Could you check a few things on this model? Use its own coordinates, in mm. A direction names the side the tool comes from. Round coordinates to 2 decimals unless told otherwise and drop trailing zeros. Write each loop counter-clockwise with the first axis right and the second up, starting at its lowest first coordinate (ties: lowest second). Pieces come first, ordered by that corner, then holes. Notation, with made-up numbers: (-7.5, 42) -> (15.5, 42) arc R11 cw to (15.5, 47) -> close; hole circle Ø10 at (17.5, 30). An arc over 180 degrees is marked (long way). Return JSON: item names as keys, results as strings.
from build123d import *

# Parameters (mm, degrees)
SKETCH_1_W      = 50
SKETCH_1_H      = 49
SKETCH_1_R      = 11.05
SKETCH_1_R_2    = 1.75
EXTRUDE_1_DEPTH = 2
EXTRUDE_2_DEPTH = 2
FILLET_2_R      = 2


with BuildPart() as part:
    # 草图1 → 凸台-拉伸1 (new body)
    with BuildSketch(Plane(origin=(0, 0, 0), x_dir=(1, 0, 0), z_dir=(0, 1, 0))):
        with Locations((-25, 0)):
            Rectangle(SKETCH_1_W, SKETCH_1_H)
        with Locations(Location((-25, 3.5, 0), (0, 0, 270))):
            Circle(SKETCH_1_R, mode=Mode.SUBTRACT)
        with Locations(Location((-40.5, 19, 0), (0, 0, 270))):
            Circle(SKETCH_1_R_2, mode=Mode.SUBTRACT)
        with Locations(Location((-9.5, 19, 0), (0, 0, 270))):
            Circle(SKETCH_1_R_2, mode=Mode.SUBTRACT)
        with Locations(Location((-9.5, -12, 0), (0, 0, 270))):
            Circle(SKETCH_1_R_2, mode=Mode.SUBTRACT)
        with Locations(Location((-40.5, -12, 0), (0, 0, 270))):
            Circle(SKETCH_1_R_2, mode=Mode.SUBTRACT)
    extrude(amount=EXTRUDE_1_DEPTH)

    # 草图2 → 凸台-拉伸2 (add)
    with BuildSketch(Plane.XY.offset(24.5)):
        Polygon((0, 0), (0, -51), (-50, -51), (-50, 0), (-50, 2), (0, 2), align=None)
        with BuildLine():
            Line((-7.9, -10), (-7.9, -40))
            ThreePointArc((-7.9, -40), (-10, -42.1), (-12.1, -40))
            Line((-12.1, -40), (-12.1, -10))
            ThreePointArc((-12.1, -10), (-10, -7.9), (-7.9, -10))
        make_face(mode=Mode.SUBTRACT)
        with BuildLine():
            Line((-37.9, -10), (-37.9, -40))
            ThreePointArc((-37.9, -40), (-40, -42.1), (-42.1, -40))
            Line((-42.1, -40), (-42.1, -10))
            ThreePointArc((-42.1, -10), (-40, -7.9), (-37.9, -10))
        make_face(mode=Mode.SUBTRACT)
    extrude(amount=EXTRUDE_2_DEPTH)

    # 圆角2
    fillet_2_edges = [part.edges().sort_by_distance(p)[0] for p in [
        (-25, 2, 26.5),
    ]]
    fillet(fillet_2_edges, radius=FILLET_2_R)


solid = part.part
1) I want a section at C-C, the plane y = -24. Please give me the cut outline in (x, z), and give its area (3 significant figures).
Return value:
{"outline": "(-50, 24.5) -> (-42.1, 24.5) -> (-42.1, 26.5) -> (-50, 26.5) -> close; (-37.9, 24.5) -> (-12.1, 24.5) -> (-12.1, 26.5) -> (-37.9, 26.5) -> close; (-7.9, 24.5) -> (0, 24.5) -> (0, 26.5) -> (-7.9, 26.5) -> close", "area": "83.2 mm²"}
2) I want a section at D-D, the plane z = 12. Please give me the cut outline in (x, y), and give its area (3 significant figures).
Return value:
{"outline": "(-50, 0) -> (-42.25, 0) -> (-42.25, 2) -> (-50, 2) -> close; (-38.75, 0) -> (-11.25, 0) -> (-11.25, 2) -> (-38.75, 2) -> close; (-7.75, 0) -> (0, 0) -> (0, 2) -> (-7.75, 2) -> close", "area": "86.0 mm²"}
3) For faces 5 (the face through (-40, -7.9, 25.5)), 6 (the face through (-25, 0, 11)), 7 (the face through (-24.65, 1.43, 25.9)), which set-ups out of +Z, -Z, +X, -X, +Y, -Y let a thin tool reach every point of the face, with its end or its side?
Return value:
{"face 5": "+Z, -Z", "face 6": "-Z, +X, -X, -Y", "face 7": "+Z, +X, -X, +Y"}
4) I want a section at B-B, the plane x = -25. Please give me the cut outline in (y, z).
Return value:
{"outline": "(-51, 24.5) -> (0, 24.5) -> (0, 7.55) -> (2, 7.55) -> (2, 24.5) arc R2 ccw to (0, 26.5) -> (-51, 26.5) -> close; (0, -24.5) -> (2, -24.5) -> (2, -14.55) -> (0, -14.55) -> close"}
5) Will these pins go through, and if not, where does the flat tip stop? pin 1 Ø2 at (x, z) = (-9.5, 12) entering from +Y; pin 2 Ø4 at (x, y) = (-28, -6.5) entering from -Z; pin 3 Ø4.5 at (x, z) = (-40.5, 12) entering from -Y.
Return value:
{"pin 1": "through", "pin 2": "z = 24.5", "pin 3": "y = 0"}
6) If I drill on probe 1 along X at (y, z) = (1, 12); probe 2 along Y at (x, z) = (-14.5, -16.5); probe 3 along Z at (x, y) = (-21.5, -23), over which ranges is the centre line in solid material (lowest first)? Write a range as [from, to].
Return value:
{"probe 1": "[-50, -42.25], [-38.75, -11.25], [-7.75, 0]", "probe 2": "[0, 2]", "probe 3": "[24.5, 26.5]"}
7) I want a section at A-A, the plane z = -3.5. Please give me the cut outline in (x, y), and give its area (3 significant figures).
Return value:
{"outline": "(-50, 0) -> (-36.05, 0) -> (-36.05, 2) -> (-50, 2) -> close; (-13.95, 0) -> (0, 0) -> (0, 2) -> (-13.95, 2) -> close", "area": "55.8 mm²"}
8) Thinking about a two-plate mould opening in Z: for faces 1 (the face through (-25, -25, 26.5)), 2 (the face through (-21.68, 0.99, 7.04)), 3 (the face through (-42.1, -25, 25)), 4 (the face through (-8.32, 0.99, -20.29)), which applies, pulls with the +Z half, pulls with the -Z half, needs draft (parallel to the pull), parting line crosses it, or undercut?
Return value:
{"face 1": "pulls with the +Z half", "face 2": "undercut", "face 3": "needs draft", "face 4": "undercut"}
